Could you check a few things on this model? Use its own coordinates, in mm. Coordinates: 2 decimals unless noted, no trailing zeros. Loops run counter-clockwise (first coordinate to the right, second up) from the corner with the lowest first, then second, coordinate; pieces in that order, holes last.
Autodesk Inventor part; units mm, degrees
ref_plane "YZ Plane" through (0, 0, 0) normal (1, 0, 0) x (0, 1, 0)
ref_plane "XZ Plane" through (0, 0, 0) normal (0, 1, 0) x (-1, 0, 0)
ref_plane "XY Plane" through (0, 0, 0) normal (0, 0, 1) x (1, 0, 0)
sketch "Sketch2" plane through (0, 0, 0) normal (1, 0, 0) x (0, 1, 0)
  line L0 (0, 0) -> (920, 0)
  line L1 (920, 0) -> (920, -50)
  line L2 (920, -50) -> (0, -50)
  line L3 (0, -50) -> (0, 0)
  line L4 (920, -50) -> (883.2713, 0) construction
  line L5 (920, 0) -> (851.9332, -50)
  line L6 (0, 0) -> (36.7287, -50)
  dimension "d28" = 920
  dimension "d29" = 50
  dimension "d31" = 36.3
  dimension "d32" = 53.7
  dimension "d36" = 53.7
extrude "Plate2" add sketch "Sketch2" along normal blind 3 contours L0 L5 L2 L6
chamfer "Corner Chamfer1" distance 3 angle 45 2 edges at (1.5, 920, 0) (1.5, 0, 0)
fillet "Corner Round1" radius 6 2 edges at (1.5, 36.7287, -50) (1.5, 851.9332, -50)
equation "\"d36\" = d32"
equation "\"d30\" = Thickness"
equation "\"BendReliefWidth\" = Thickness"
equation "\"BendReliefDepth\" = 0.5 * Thickness"
equation "\"CornerReliefSize\" = 4 * Thickness"
equation "\"MinimumRemnant\" = 2 * Thickness"
equation "\"TransitionRadius\" = BendRadius"
equation "\"JacobiRadiusSize\" = BendRadius"
equation "\"GapSize\" = Thickness"
properties part number "MSC 0691 stringer cone" material "Stainless Steel"
(1) Imagine slicing it at A-A, the plane x = 1.75. Write out the boundary of the cut face in (y, z).
Answers:
outline: (1.78, -2.42) - (34.93, -47.55) arc R6 ccw to (39.77, -50) - (849.97, -50) arc R6 ccw to (853.52, -48.84) - (917.58, -1.78) - (917, 0) - (3, 0) - close
(2) I need wall thicknesses on probe 1 along Y at (x, z) = (2.05, -28); probe 2 along Y at (x, z) = (2.5, -9). Which ranges of each line are inside material? Lowest first, please.
Answers:
probe 1: y = 20.57 to 881.88
probe 2: y = 6.61 to 907.75
(3) Imagine slicing it at B-B, the plane z = -23.5. Write out the boundary of the cut face in (x, y).
Answers:
outline: (0, 17.26) - (3, 17.26) - (3, 888.01) - (0, 888.01) - close
(4) For pin 1 (1.5 mm diameter, centred on x = 1.5, z = -6, fed in from -Y); pin 2 (10 mm diameter, centred on y = 305, z = -11, fed in from -X); pin 3 (1 mm diameter, centred on x = 1, z = -35, fed in from +Y), each with a flat end and sliding along its axis, tell me the tip position at first contact or that it passes through.
Answers:
pin 1: stops at y = 3.86
pin 2: stops at x = 0
pin 3: stops at y = 873.03
